from build123d import *

# Parameters (mm, degrees)
SKETCH1_W           = 210
SKETCH1_H           = 164
BOSS_EXTRUDE1_DEPTH = 5
SKETCH2_W           = 164
SKETCH2_H           = 210
SKETCH2_W_2         = 154
SKETCH2_H_2         = 200
BOSS_EXTRUDE2_DEPTH = 12
SKETCH3_R           = 2
CUT_EXTRUDE1_DEPTH  = 159


with BuildPart() as part:
    # Sketch1 → Boss-Extrude1 (new body)
    with BuildSketch(Plane(origin=(0, 0, 0), x_dir=(0, 1, 0), z_dir=(0, 0, 1))):
        Rectangle(SKETCH1_W, SKETCH1_H)
    extrude(amount=BOSS_EXTRUDE1_DEPTH)

    # Sketch2 → Boss-Extrude2 (add)
    with BuildSketch(Plane.XY.offset(5)):
        Rectangle(SKETCH2_W, SKETCH2_H)
        Rectangle(SKETCH2_W_2, SKETCH2_H_2, mode=Mode.SUBTRACT)
    extrude(amount=BOSS_EXTRUDE2_DEPTH)

    # Sketch3 → Cut-Extrude1 (cut)
    with BuildSketch(Plane(origin=(77, 0, 0), x_dir=(0, -1, 0), z_dir=(-1, 0, 0))):
        with Locations(Location((-79.5, 11, 0), (0, 0, 270))):
            Circle(SKETCH3_R)
    extrude(amount=CUT_EXTRUDE1_DEPTH, mode=Mode.SUBTRACT)


solid = part.part
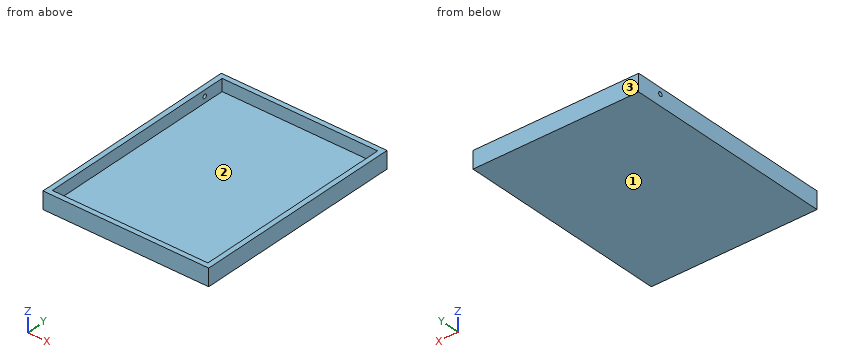
The listing builds one solid part. Answer for the finished solid, in the listing's coordinates (mm). Face numbers are marked on the shaded views. Give positions to 0.01 mm unless a question says otherwise; leave off trailing zeros. Write each loop counter-clockwise with the first axis right and the second up, starting at its lowest first coordinate (ties: lowest second). Pieces come first, ordered by that corner, then holes.
1) Section A-A (x = -48.5) is taken. Write down the section's boundary in (y, z).
2) Section B-B (y = 56) is taken. Write down the section's boundary in (x, z), and give its area (3 significant figures).
3) Given P1, Ø5, axis at x = -11.5, y = -47.5, coming from the -Z side; P2, Ø3.5, axis at y = 79.5, z = 11, coming from the -X side; P3, Ø6, axis at x = -14, y = 14.5, coming from the +Z side, each flat-ended and moving along its own axis, determine where each tip first touches the part or whether it passes through.
4) Find the intervals of material crossed by L1, parallel to Y at x = 46.5, z = 8.25; L2, parallel to Z at x = -79.7, y = 79.5; L3, parallel to X at y = 41, z = 10.75, in increasing order.
5) For a pull along Y with two mould halves and no side action, classify the marked faces 1, 2 and 3 as pulls with the +Y half, pulls with the -Y half, needs draft (parallel to the pull), parting line crosses it, or undercut.
Response:
1. outline: (-105, 0) - (105, 0) - (105, 17) - (100, 17) - (100, 5) - (-100, 5) - (-100, 17) - (-105, 17) - close
2. outline: (-82, 0) - (82, 0) - (82, 17) - (77, 17) - (77, 5) - (-77, 5) - (-77, 17) - (-82, 17) - close
2. area: 940 mm2
3. P1: stops at z = 0
3. P2: stops at x = 77
3. P3: stops at z = 5
4. L1: y = -105 to -100, 100 to 105
4. L2: z = 0 to 9, 13 to 17
4. L3: x = -82 to -77, 77 to 82
5. face 1: needs draft
5. face 2: undercut
5. face 3: pulls with the +Y half
